Geometry check sheet. Reference: the model listing, model coordinates, mm. A direction names the side the tool comes from. Coordinates: 2 decimals unless noted, no trailing zeros. Loops run counter-clockwise (first coordinate to the right, second up) from the corner with the lowest first, then second, coordinate; pieces in that order, holes last.
Autodesk Inventor part; units mm, degrees
ref_plane "Work Plane2" through (6.8027, 0, 0) normal (1, 0, 0) x (0, 1, 0)
ref_plane "YZ 0" through (6.803, 0, 0) normal (1, 0, 0) x (0, 1, 0)
ref_plane "XY 0" through (0, 0, -11.25) normal (0, 0, 1) x (1, 0, 0)
sketch "Sketch1" plane through (0, 0, 0) normal (0, 1, 0) x (-1, 0, 0)
  line L0 (43.1973, 3.7398) -> (-56.8027, 3.7398)
  line L1 (-56.8027, 3.7398) -> (-56.8027, -26.2602)
  line L2 (43.1973, 3.7398) -> (43.1973, -26.2602)
  line L3 (-21.8027, -26.2602) -> (8.1973, -26.2602)
  line L4 (43.1973, -26.2602) -> (8.1973, -26.2602)
  line L5 (-21.8027, -26.2602) -> (-56.8027, -26.2602)
  line L6 (-21.8027, 3.7398) -> (8.1973, 3.7398)
  point P0 (0, 0)
  dimension "d2" = 100
  dimension "d6" = 30
extrude "Extrusion1" add sketch "Sketch1" along normal blind 5
sketch "Sketch4" plane through (0, 5, 0) normal (0, 1, 0) x (1, 0, 0)
  circle A0 centre (-36.6973, 2.7602) radius 1.75
  circle A1 centre (-36.6973, 19.7602) radius 1.75
  circle A2 centre (14.0028, 2.7602) radius 1.75
  circle A3 centre (14.0028, 19.7602) radius 1.75
  point P0 (0, 0)
extrude "Extrusion3" cut sketch "Sketch4" against normal through all
sketch "Sketch5" plane through (0, 0, 0) normal (0, -1, 0) x (1, 0, 0)
  circle A0 centre (41.8754, -14.1565) radius 1.5
  circle A1 centre (48.1213, -10.8415) radius 1.5
  circle A2 centre (44.8063, -4.5956) radius 1.5
  circle A3 centre (38.5604, -7.9106) radius 1.5
  line L0 (44.8063, -4.5956) -> (48.1213, -10.8415) construction
  line L1 (48.1213, -10.8415) -> (41.8754, -14.1565) construction
  line L2 (41.8754, -14.1565) -> (38.5604, -7.9106) construction
  line L3 (38.5604, -7.9106) -> (44.8063, -4.5956) construction
  line L4 (44.8063, -4.5956) -> (41.8754, -14.1565) construction
  line L5 (48.1213, -10.8415) -> (38.5604, -7.9106) construction
  line L6 (43.3409, -9.376) -> (52.1686, -4.6925)
  point P0 (0, 0)
  dimension "d47" = 3
  dimension "d48" = 3
  dimension "d49" = 3
  dimension "d50" = 3
  dimension "d51" = 3.315
  dimension "d52" = 3.315
  dimension "d53" = 7.0711
  dimension "d54" = 7.0711
  dimension "d55" = 7.0711
  dimension "d56" = 7.0711
extrude "Extrusion4" cut sketch "Sketch5" against normal up to next
sketch "Sketch6" plane through (0, 0, 0) normal (0, -1, 0) x (1, 0, 0)
  circle A0 centre (6.7527, 80.0276) radius 4.235
  circle A1 centre (6.7527, 80.0276) radius 4.8512
  point P0 (0, 0)
  dimension "d19" = 0.6162
sketch "Sketch7" plane through (-43.1973, 0, 3.7398) normal (0, 0, 1) x (1, 0, 0)
  line L0 (0, 0) -> (100, 0)
  line L1 (100, 0) -> (100, 5)
  line L2 (0, 5) -> (100, 5)
  line L3 (0, 0) -> (0, 5)
  line L4 (65, 0) -> (35, 0)
  line L5 (35, 0) -> (35, 5)
  line L6 (35, 5) -> (65, 5)
  line L7 (65, 5) -> (65, 0)
  line L8 (65, 0) -> (35, 5) construction
  line L9 (35, 0) -> (65, 5) construction
  point P0 (43.1973, 0)
  point P1 (50, 2.5)
  dimension "d22" = 30
  dimension "d23" = 5
  dimension "d24" = 6.8027
  dimension "d57" = 0
ref_plane "Work Plane2" through (6.8027, 0, 0) normal (1, 0, 0) x (0, 1, 0)
sketch "Sketch9" plane through (6.8027, 0, 0) normal (1, 0, 0) x (0, 1, 0)
  line L0 (2.5, 3.7398) -> (2.5, 8.7398)
  line L1 (2.5, 3.7398) -> (7.5, 3.7398) construction
  line L2 (2.5, 8.7398) -> (27.5, 8.7398)
  line L3 (27.5, 8.7398) -> (27.5, 88.7398)
  point P0 (0, 0)
  dimension "d26" = 5
  dimension "d27" = 90
  dimension "d28" = 25
  dimension "d29" = 80
sweep "Sweep1" add profiles "Sketch7" path "Sketch9" contours L5 L2 L7 L0
ref_plane "YZ 0" through (6.803, 0, 0) normal (1, 0, 0) x (0, 1, 0)
ref_plane "XY 0" through (0, 0, -11.25) normal (0, 0, 1) x (1, 0, 0)
sketch "Sketch12" plane through (-8.1973, 25, 11.2398) normal (0, -1, 0) x (1, 0, 0)
  circle A0 centre (15.0003, 42.485) radius 1.11
  point P0 (8.1973, -11.2398)
extrude "Extrusion8" cut sketch "Sketch12" against normal up to next
sketch "Sketch13" plane through (-8.1973, 30, 6.2398) normal (0, 1, 0) x (1, 0, 0)
  circle A0 centre (15.0003, -45.985) radius 1.4
  point P0 (8.1973, 6.2398)
extrude "Extrusion9" cut sketch "Sketch13" against normal up to next
sketch "Sketch15" plane through (-8.1973, 30, 6.2398) normal (0, 1, 0) x (1, 0, 0)
  circle A0 centre (15, -40) radius 4.5
  point P0 (8.1973, 6.2398)
  dimension "d40" = 9
extrude "Extrusion10" cut sketch "Sketch15" against normal up to next
sketch "Sketch16" plane through (-8.1973, 25, 11.2398) normal (0, -1, 0) x (1, 0, 0)
  circle A0 centre (15, 42.5) radius 12
  line L0 (30, 0) -> (30, 77.5)
  line L1 (0, 0) -> (0, 77.5)
  line L2 (30, 77.5) -> (0, 77.5)
  line L3 (0, 77.5) -> (0, 57.5)
  line L4 (0, 57.5) -> (30, 57.5)
  line L5 (30, 57.5) -> (30, 77.5)
  point P0 (8.1973, -11.2398)
  point P1 (15, 57.5)
  dimension "d43" = 15
  dimension "d44" = 15
extrude "Extrusion11" cut sketch "Sketch16" against normal up to next contours L4 L1 L2 L0
sketch "Sketch17" plane through (-8.1973, 30, 6.2398) normal (0, 1, 0) x (1, 0, 0)
  circle A0 centre (8.9896, -46.0153) radius 1.25
  circle A1 centre (8.9896, -33.9945) radius 1.25
  circle A2 centre (21.0104, -46.0153) radius 1.25
  circle A3 centre (21.0104, -33.9945) radius 1.25
  line L0 (8.9896, -46.0153) -> (8.9896, -33.9945) construction
  line L1 (8.9896, -33.9945) -> (21.0104, -33.9945) construction
  line L2 (21.0104, -33.9945) -> (21.0104, -46.0153) construction
  line L3 (21.0104, -46.0153) -> (8.9896, -46.0153) construction
  line L4 (21.0104, -33.9945) -> (8.9896, -46.0153) construction
  line L5 (8.9896, -33.9945) -> (21.0104, -46.0153) construction
  line L6 (0, -62.5) -> (30, -62.5) construction
  line L7 (0, 0) -> (0, -62.5) construction
  line L8 (30, 0) -> (30, -62.5) construction
  point P0 (8.1973, 6.2398)
  dimension "d64" = 12.0208
  dimension "d65" = 12.0208
  dimension "d66" = 12.0208
  dimension "d67" = 12.0208
  dimension "d68" = 17
  dimension "d69" = 17
  dimension "d70" = 2.5
  dimension "d71" = 2.5
  dimension "d72" = 2.5
  dimension "d73" = 2.5
extrude "Extrusion12" cut sketch "Sketch17" against normal up to next
sketch "Sketch18" plane through (6.803, 0, 0) normal (1, 0, 0) x (0, 1, 0)
  line L0 (25, 11.2398) -> (15, 11.2398)
  line L1 (0, 11.2398) -> (25, 11.2398)
  line L2 (25, 11.2398) -> (25, 21.2398)
  line L3 (25, 11.2398) -> (25, 68.7398)
  line L4 (25, 21.2398) -> (15, 11.2398)
  point P0 (0, 0)
  dimension "d76" = 10
  dimension "d79" = 10
extrude "Extrusion13" add sketch "Sketch18" along normal mid plane 30
sketch "Sketch19" plane through (6.803, 0, 0) normal (1, 0, 0) x (0, 1, 0)
  line L0 (5, 6.2398) -> (7.5, 6.2398)
  line L1 (5, 6.2398) -> (30, 6.2398)
  line L2 (5, 6.2398) -> (7.5, 6.2398) construction
  line L3 (7.5, 6.2398) -> (5, 3.7398)
  line L4 (5, 3.7398) -> (5, 6.2398)
  point P0 (0, 0)
  dimension "d80" = 2.5
  dimension "d81" = 0
  dimension "d82" = 45
extrude "Extrusion14" add sketch "Sketch19" along normal mid plane 30
sketch "Sketch20" plane through (-8.1973, 30, 6.2398) normal (0, 1, 0) x (1, 0, 0)
  circle A0 centre (15, -40) radius 4.5
  arc A1 (15.9875, -46.9776) -> (14.013, -46.9776) centre (15.0003, -45.985) ccw
  arc A2 (14.013, -46.9776) -> (15.9875, -46.9776) centre (15.0003, -47.485) ccw
  point P0 (8.1973, 6.2398)
extrude "Extrusion15" add sketch "Sketch20" against normal blind 5 contours A2 A1
sketch "Sketch21" plane through (-8.1973, 25, 68.7398) normal (0, -1, 0) x (1, 0, 0)
  line L0 (30, -47.5) -> (30, 0)
  line L1 (0, 0) -> (30, 0)
  line L2 (30, 0) -> (30, -8)
  line L3 (30, -8) -> (0, -8)
  line L4 (0, -8) -> (0, 0)
  point P0 (8.1973, -68.7398)
extrude "Extrusion16" cut sketch "Sketch21" against normal through all
equation "\"d71\" = d70"
equation "\"d72\" = d70"
equation "\"d73\" = d70"
properties part number "DudukanExt"
1) Material ranges on probe 1 along X at (y, z) = (28, 40.5); probe 2 along Y at (x, z) = (18, -2); probe 3 along X at (y, z) = (8, 8), recorded low to high.
Data:
probe 1: x = -8.2 to -0.43, 2.01 to 11.59, 14.03 to 21.8
probe 2: y = 0 to 5
probe 3: x = -8.2 to 21.8
2) Section check A-A on y = 28. Record the cut outline in (x, z).
Data:
outline: (-8.2, 6.24) - (21.8, 6.24) - (21.8, 60.74) - (-8.2, 60.74) - close; hole circle Ø2.5 at (0.79, 40.23); hole circle Ø2.5 at (0.79, 52.26); hole circle Ø9 at (6.8, 46.24); hole circle Ø2.5 at (12.81, 40.23); hole circle Ø2.5 at (12.81, 52.26)
3) Section check C-C on z = 49. Record the cut outline in (x, y), and give its area (3 significant figures).
Data:
outline: (-8.2, 25) - (3.25, 25) - (3.25, 30) - (-8.2, 30) - close; (10.36, 25) - (21.8, 25) - (21.8, 30) - (10.36, 30) - close
area: 114 mm2
4) Section check B-B on x = -6.5. Record the cut outline in (y, z), and give its area (3 significant figures).
Data:
outline: (0, -26.26) - (5, -26.26) - (5, 3.74) - (7.5, 6.24) - (30, 6.24) - (30, 60.74) - (25, 60.74) - (25, 21.24) - (15, 11.24) - (0, 11.24) - close
area: 613 mm2
5) Depth check by flat-ended pin: pin 1 (1.8 mm diameter, centred on x = 48.12, z = -10.84, fed in from -Y); pin 2 (5 mm diameter, centred on x = 5, y = 18.5, fed in from -Z); pin 3 (8 mm diameter, centred on y = 17.5, z = 17.5, fed in from -X); pin 4 (5 mm diameter, centred on y = 20, z = 16, fed in from +X). Enter the tip coordinate at first touch or a pass-through.
Data:
pin 1: passes through
pin 2: stops at z = 6.24
pin 3: stops at x = -8.2
pin 4: stops at x = 21.8
6) Mould release check, pull along Z, two halves, no side actions. Record for faces 4 (the flat face through (21.803, 6, 5)), 5 (the cylindrical face through (40.685, 2.465, -15.069)), 6 (the flat face through (6, 2, -26.26)): +Z half, -Z half, draft (parallel to the pull), parting line (faces both ways), or undercut.
Data:
face 4: draft
face 5: undercut
face 6: -Z half
7) Access from +Z, -Z, +X, -X, +Y, -Y to the whole of each face (thin tool, end or side, straight path). Record for faces 1 (the cylindrical face through (9.222, 27.535, 42.445)), 2 (the flat face through (-26, 2, 3.74)), 3 (the flat face through (7, 7, 11.24)).
Data:
face 1: +Y, -Y
face 2: +Z, -X, +Y, -Y
face 3: +Z, +X, -X, -Y
